Can you work these out from the model? Positions are in its coordinate system, mm. A direction names the side the tool comes from. Coordinates: 2 decimals unless noted, no trailing zeros. Loops run counter-clockwise (first coordinate to the right, second up) from the corner with the lowest first, then second, coordinate; pieces in that order, holes last. Notation, with made-up numbers: M 52,-14 L 75,-14 A10 ccw 75,-5 Z; hole C 24.25,43.5 d8. An arc over 180 degrees is marked long. Return JSON: item names as keys, results as strings. Group by question number.
```python
from build123d import *

# Parameters (mm, degrees)
SKETCH1_W          = 25
SKETCH1_H          = 25
SKETCH1_R          = 1.55
EXTRUDE1_DEPTH     = 15
SKETCH2_R          = 7
CUT_EXTRUDE1_DEPTH = 10
SKETCH3_R          = 3.175
CUT_EXTRUDE2_DEPTH = 39.405728739
SKETCH4_R          = 3.175
CUT_EXTRUDE3_DEPTH = 10
SKETCH7_R          = 8.65
CUT_EXTRUDE4_DEPTH = 1.3


with BuildPart() as part:
    # Sketch1 → Extrude1 (new body)
    with BuildSketch(Plane(origin=(0, 0, 0), x_dir=(0, 0, -1), z_dir=(1, 0, 0))):
        with Locations((12.5, 12.5)):
            Rectangle(SKETCH1_W, SKETCH1_H)
        with Locations((4, 4)):
            Circle(SKETCH1_R, mode=Mode.SUBTRACT)
        with Locations((4, 21)):
            Circle(SKETCH1_R, mode=Mode.SUBTRACT)
        with Locations((21, 21)):
            Circle(SKETCH1_R, mode=Mode.SUBTRACT)
        with Locations((21, 4)):
            Circle(SKETCH1_R, mode=Mode.SUBTRACT)
    extrude(amount=-EXTRUDE1_DEPTH)

    # Sketch2 → Cut-Extrude1 (cut)
    with BuildSketch(Plane(origin=(0, 0, 0), x_dir=(0, 0, -1), z_dir=(1, 0, 0))):
        with Locations((12.5, 12.5)):
            Circle(SKETCH2_R)
    extrude(amount=-CUT_EXTRUDE1_DEPTH, mode=Mode.SUBTRACT)

    # Sketch3 → Cut-Extrude2 (cut, through all)
    with BuildSketch(Plane(origin=(0, 0, 0), x_dir=(0, 0, -1), z_dir=(1, 0, 0))):
        with Locations((12.5, 12.5)):
            Circle(SKETCH3_R)
    extrude(amount=-CUT_EXTRUDE2_DEPTH, mode=Mode.SUBTRACT)

    # Sketch4 → Cut-Extrude3 (cut)
    with BuildSketch(Plane(origin=(0, 25, 0), x_dir=(1, 0, 0), z_dir=(0, 1, 0))):
        with Locations(Location((-6, 12.5, 0), (0, 0, 270))):
            Circle(SKETCH4_R)
    extrude(amount=-CUT_EXTRUDE3_DEPTH, mode=Mode.SUBTRACT)

    # Sketch7 → Cut-Extrude4 (cut)
    with BuildSketch(Plane(origin=(0, 0, 0), x_dir=(0, 0, -1), z_dir=(1, 0, 0))):
        with Locations((12.5, 12.5)):
            Circle(SKETCH7_R)
    extrude(amount=-CUT_EXTRUDE4_DEPTH, mode=Mode.SUBTRACT)


solid = part.part
```
1) Suppose I cut it at D-D, the plane x = -11. List the corners of the cut face in (y, z) for me (3 decimals).
2) For faces 1 (the face through (-10, 9, -14)), 2 (the face through (-15, 15, -10)), which set-ups out of +Z, -Z, +X, -X, +Y, -Y let a thin tool reach every point of the face, with its end or its side?
3) Suppose I cut it at B-B, the plane x = -6. List the corners of the cut face in (y, z) for me (3 decimals).
4) For pin 1 (1 mm diameter, centred on y = 17, z = -10, fed in from +X), with a flat end and sliding along its axis, tell me the tip position at first contact or that it passes through.
5) Suppose I cut it at C-C, the plane y = 3.5. List the corners of the cut face in (x, z) for me, then the cut area to 3 significant figures.
6) If we mould it in two halves opening along Y, with no side actions, what happens to faces 3 (the face through (-5.59, 6.29, -15.73)), 4 (the face through (-9, 25, -10)), 5 (the face through (-5.86, 21.91, -15.67)), 6 (the face through (-7.395, 22.537, -20.798))? For each: +Y half, -Y half, draft (parallel to the pull), parting line (faces both ways), or undercut.
7) Suppose I cut it at A-A, the plane z = -12.5. List the corners of the cut face in (x, y) for me (3 decimals), then the cut area to 3 significant figures.
8) If I drill on line 1 (Y direction, x = -11.25, z = -4); line 2 (Y direction, x = -1.5, z = -22.25); line 3 (X direction, y = 13.75, z = -17.5), over which ranges is the centre line in solid material (lowest first)? Write a range as from..to.
Returned:
{
 "1": {"outline": "M 0,-25 L 25,-25 L 25,0 L 0,0 Z; hole C 4,-21 d3.1; hole C 4,-4 d3.1; hole C 12.5,-12.5 d6.35; hole C 21,-21 d3.1; hole C 21,-4 d3.1"},
 "2": {"face 1": "+X", "face 2": "+Z, -Z, -X, +Y, -Y"},
 "3": {"outline": "M 0,-25 L 25,-25 L 25,-15.675 L 18.739,-15.675 A7 cw long 18.739,-9.325 L 25,-9.325 L 25,0 L 0,0 Z; hole C 4,-21 d3.1; hole C 4,-4 d3.1; hole C 21,-21 d3.1; hole C 21,-4 d3.1"},
 "4": {"pin 1": "stops at x = -10"},
 "5": {"outline": "M -15,-25 L 0,-25 L 0,-22.47 L -15,-22.47 Z; M -15,-19.53 L 0,-19.53 L 0,-5.47 L -15,-5.47 Z; M -15,-2.53 L 0,-2.53 L 0,0 L -15,0 Z", "area": "287 mm²"},
 "6": {"face 3": "undercut", "face 4": "+Y half", "face 5": "draft", "face 6": "undercut"},
 "7": {"outline": "M -15,0 L 0,0 L 0,3.85 L -1.3,3.85 L -1.3,5.5 L -10,5.5 L -10,9.325 L -15,9.325 Z; M -15,15.675 L -10,15.675 L -10,19.5 L -9.175,19.5 L -9.175,25 L -15,25 Z; M -2.825,19.5 L -1.3,19.5 L -1.3,21.15 L 0,21.15 L 0,25 L -2.825,25 Z", "area": "164 mm²"},
 "8": {"line 1": "y = 0..2.45, 5.55..19.45, 22.55..25", "line 2": "y = 0..3.08, 4.92..20.08, 21.92..25", "line 3": "x = -15..-10"}
}
